Part model, mm, in its own coordinate system. Face numbers are marked on the shaded views. A direction names the side the tool comes from. Give positions to 0.01 mm unless a question says otherwise; leave off trailing zeros. Order: outer loops, then holes, each group sorted by start corner. A loop starts at its lowest first (then second) coordinate and runs counter-clockwise, first axis right, second up.
from build123d import *

# Parameters (mm, degrees)
SKETCH1_R               = 1.3589
EXTRUDE1_DEPTH          = 2.54
EXTRUDE2_DEPTH          = 7.366
SKETCH3_R               = 4.0259
CUT_EXTRUDE1_DEPTH      = 19.513485712
CUT_EXTRUDE2_DEPTH      = 19.513485712
CUT_EXTRUDE2_DEPTH_BACK = 7.366
SKETCH4_R               = 1.27


with BuildPart() as part:
    # Sketch1 → Extrude1 (new body)
    with BuildSketch(Plane.XY):
        with BuildLine():
            ThreePointArc((7.9248, 2.2987), (3.603126127, 4.22759635), (2.153092948, 8.732583583))
            ThreePointArc((2.153092948, 8.732583583), (2.211696246, 9.137709934), (2.2987, 9.5377))
            ThreePointArc((2.2987, 9.5377), (0, 11.8364), (-2.2987, 9.5377))
            ThreePointArc((-2.2987, 9.5377), (-3.870608713, 4.953593702), (-7.9248, 2.2987))
            ThreePointArc((-7.9248, 2.2987), (-10.2235, 0), (-7.9248, -2.2987))
            ThreePointArc((-7.9248, -2.2987), (-3.603126127, -4.22759635), (-2.153092948, -8.732583583))
            ThreePointArc((-2.153092948, -8.732583583), (-2.211696246, -9.137709934), (-2.2987, -9.5377))
            ThreePointArc((-2.2987, -9.5377), (0, -11.8364), (2.2987, -9.5377))
            ThreePointArc((2.2987, -9.5377), (3.870608713, -4.953593702), (7.9248, -2.2987))
            ThreePointArc((7.9248, -2.2987), (10.2235, 0), (7.9248, 2.2987))
        make_face()
        with Locations((0, -9.5377)):
            Circle(SKETCH1_R, mode=Mode.SUBTRACT)
        with Locations((-7.9248, 0)):
            Circle(SKETCH1_R, mode=Mode.SUBTRACT)
        with Locations((7.9248, 0)):
            Circle(SKETCH1_R, mode=Mode.SUBTRACT)
        with Locations((0, 9.5377)):
            Circle(SKETCH1_R, mode=Mode.SUBTRACT)
    extrude(amount=EXTRUDE1_DEPTH)

    # Sketch2 → Extrude2 (add)
    with BuildSketch(Plane.XY.offset(2.54)):
        with BuildLine():
            ThreePointArc((0, 6.990319603), (-5.303505549, 0), (0, -6.990319603))
            ThreePointArc((0, -6.990319603), (5.303505549, 0), (0, 6.990319603))
        make_face()
    extrude(amount=EXTRUDE2_DEPTH)

    # Sketch3 → Cut-Extrude1 (cut, through all)
    with BuildSketch(Plane.XY.offset(9.906)):
        Circle(SKETCH3_R)
    extrude(amount=-CUT_EXTRUDE1_DEPTH, mode=Mode.SUBTRACT)

    # Sketch4 → Cut-Extrude2 (cut, two sides: drawn at the far end of the back side and taken through both)
    with BuildSketch(Plane(origin=(0, 0, 0), x_dir=(1, 0, 0), z_dir=(0, 1, 0)).offset(-CUT_EXTRUDE2_DEPTH_BACK)):
        with Locations(Location((0, -5.461, 0), (0, 0, 270))):
            Circle(SKETCH4_R)
    extrude(amount=CUT_EXTRUDE2_DEPTH + CUT_EXTRUDE2_DEPTH_BACK, mode=Mode.SUBTRACT)


solid = part.part
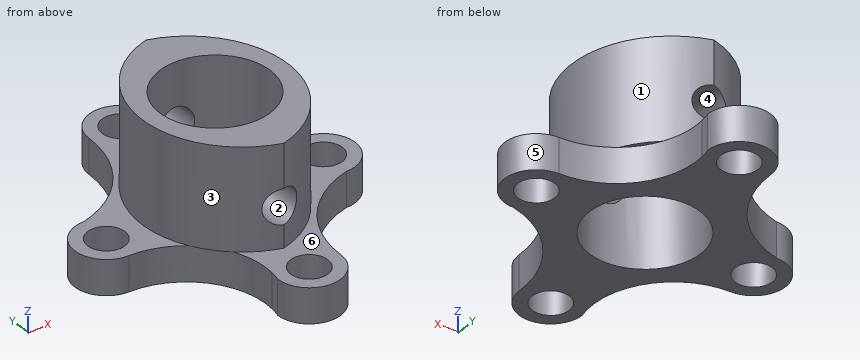
Item 1: Which spindle directions (+Z, -Z, +X, -X, +Y, -Y) get a long thin tool onto all of the face, cutting with end or side? Do the marked faces 1, 2 and 3. Say none if no direction does.
Item 2: Pull direction Z, two halves, no side cores. Call the marked faces 4, 5 and 6: released by +Z, released by -Z, zero draft, split by the parting line, or undercut.
Item 3: Band-saw the part on C-C on z = 4.75. List the corners of the cut face in (x, y).
Item 4: Drill centre lines: probe 1 along Y at (x, z) = (0, 0.95); probe 2 along Z at (x, y) = (0, -5.25); probe 3 along Y at (x, z) = (-1.5, 4.75). Where is each one in solid material? Low to high.
Item 5: Band-saw the part on D-D on y = -3. List the corners of the cut face in (x, z), plus the area to 3 significant figures.
Item 6: Drop flat-ended pins along their axis: P1, Ø3.5, axis at x = -7.92, y = 0, coming from the +Z side; P2, Ø1.4, axis at x = -4, y = -5, coming from the -Z side; P3, Ø1.5, axis at y = 3, z = 8.5, coming from the +X side. Give the stop position or say it passes through.
Item 7: Band-saw the part on A-A on y = 0. List the corners of the cut face in (x, z), plus the area to 3 significant figures.
Item 8: Band-saw the part on B-B on x = -3.25. List the corners of the cut face in (y, z), plus the area to 3 significant figures.
Working result:
1. face 1: +Z, +X
1. face 2: +Y, -Y
1. face 3: +Z, -X
2. face 4: undercut
2. face 5: zero draft
2. face 6: released by +Z
3. outline: (-1.05, -6.61) - (-1.05, -3.89) arc R4.03 cw to (-1.05, 3.89) - (-1.05, 6.61) arc R7.26 ccw to start; (1.05, -6.61) arc R7.26 ccw to (1.05, 6.61) - (1.05, 3.89) arc R4.03 cw to (1.05, -3.89) - close
4. probe 1: y = -11.84 to -10.9, -8.18 to -4.03, 4.03 to 8.18, 10.9 to 11.84
4. probe 2: z = 0 to 4.19, 6.73 to 9.91
4. probe 3: y = -6.38 to -3.74, 3.74 to 6.38
5. outline: (-5.16, 0) - (-2.68, 0) - (-2.68, 9.91) - (-4.65, 9.91) - (-4.65, 2.54) - (-5.16, 2.54) - close; (2.68, 0) - (6.15, 0) - (6.15, 2.54) - (4.65, 2.54) - (4.65, 9.91) - (2.68, 9.91) - close
5. area: 44.1 mm2
6. P1: stops at z = 2.54
6. P2: stops at z = 2.54
6. P3: stops at x = 4.95
7. outline: (-10.22, 0) - (-9.28, 0) - (-9.28, 2.54) - (-10.22, 2.54) - close; (-6.57, 0) - (-4.03, 0) - (-4.03, 9.91) - (-5.3, 9.91) - (-5.3, 2.54) - (-6.57, 2.54) - close; (4.03, 0) - (6.57, 0) - (6.57, 2.54) - (5.3, 2.54) - (5.3, 9.91) - (4.03, 9.91) - close; (9.28, 0) - (10.22, 0) - (10.22, 2.54) - (9.28, 2.54) - close
7. area: 36.5 mm2
8. outline: (-5.06, 2.54) - (-4.66, 2.54) - (-4.66, 0) - (-2.38, 0) - (-2.38, 9.91) - (-5.06, 9.91) - close; (2.38, 0) - (5.89, 0) - (5.89, 2.54) - (5.06, 2.54) - (5.06, 9.91) - (2.38, 9.91) - close
8. area: 54.3 mm2
